Read the model definition and answer for the solid it produces. Units are mm, in the model's axes. A direction names the side the tool comes from. Give positions to 0.01 mm unless a question says otherwise; leave off trailing zeros. Loops run counter-clockwise (first coordinate to the right, second up) from the corner with the lowest first, then second, coordinate; pieces in that order, holes last. Notation, with made-up numbers: (-14.5, 3.5) - (33.5, 3.5) arc R35 ccw to (33.5, 39.5) - close; hole circle Ø7 at (-2.75, -34.5). An arc over 180 degrees is marked (long way). Write item = value, one per line. Start each with the question number.
from build123d import *

# Parameters (mm, degrees)
F1_DEPTH      = 17.5
F1_DEPTH_BACK = 17.5
F2_R          = 2.6
F3_DEPTH      = 10.001
F4_R          = 2.6
F5_DEPTH      = 10.001


with BuildPart() as f1:
    # F0 (on Right) → F1 (new body, two sides)
    with BuildSketch(Plane.YZ) as f1_sk:
        Polygon((-30, 0), (0, 0), (0, 30), (-10, 30), (-10, 10), (-30, 10), align=None)
    extrude(amount=F1_DEPTH)
    extrude(f1_sk.sketch, amount=-F1_DEPTH_BACK)

    # F2 (on face) → F3 (cut, through all)
    with BuildSketch(Plane.XZ.offset(10)):
        with Locations((-7.5, 20)):
            Circle(F2_R)
        with Locations((7.5, 20)):
            Circle(F2_R)
    extrude(amount=-F3_DEPTH, mode=Mode.SUBTRACT)

    # F4 (on face) → F5 (cut, through all)
    with BuildSketch(Plane.XY.offset(10)):
        with Locations((-7.5, -20)):
            Circle(F4_R)
        with Locations((7.5, -20)):
            Circle(F4_R)
    extrude(amount=-F5_DEPTH, mode=Mode.SUBTRACT)


solid = f1.part
1. A cutting plane is placed at B-B on z = 20. Give the vertices of the cut face in (x, y).
2. Given P1, Ø8.5, axis at x = 7.5, y = -20, coming from the +Z side; P2, Ø6, axis at x = 7.5, z = 20, coming from the -Y side, each flat-ended and moving along its own axis, determine where each tip first touches the part or whether it passes through.
3. For a pull along X with two mould halves and no side action, classify faces 1 (the cylindrical face through (-7.838, -5.07, 22.578)), 2 (the flat face through (-17.5, -9, 12)), 3 (the flat face through (0, -5, 30)), 4 (the cylindrical face through (9.98, -19.22, 5.07)) as released by +X, released by -X, zero draft, split by the parting line, or undercut.
4. A cutting plane is placed at C-C on y = -20. Give the vertices of the cut face in (x, z), and give its area (3 significant figures).
5. A cutting plane is placed at A-A on x = 7.5. Give the vertices of the cut face in (y, z), and give its area (3 significant figures).
6. A tool of negligible diameter and unlimited length cuts with its end or side. For faces 5 (the flat face through (0, -20, 10)), 6 (the flat face through (0, 0, 15)), from which of +Z, -Z, +X, -X, +Y, -Y can it reach the whole face along a straight path? Write none if from no direction.
7. Consider line 1 along Z through (x, y) = (12, -11); line 2 along Y through (x, z) = (10, 25.5); line 3 along Z through (x, y) = (-7.5, -7). Determine where each line is inside the solid, lowest interval first. Write a range as [from, to].
8. A cutting plane is placed at D-D on z = 2.5. Give the vertices of the cut face in (x, y), and give its area (3 significant figures).
Reply:
q1.outline = (-17.5, -10) - (-10.1, -10) - (-10.1, 0) - (-17.5, 0) - close; (-4.9, -10) - (4.9, -10) - (4.9, 0) - (-4.9, 0) - close; (10.1, -10) - (17.5, -10) - (17.5, 0) - (10.1, 0) - close
q2.P1 = 10
q2.P2 = -10
q3.face_1 = undercut
q3.face_2 = released by -X
q3.face_3 = zero draft
q3.face_4 = undercut
q4.outline = (-17.5, 0) - (-10.1, 0) - (-10.1, 10) - (-17.5, 10) - close; (-4.9, 0) - (4.9, 0) - (4.9, 10) - (-4.9, 10) - close; (10.1, 0) - (17.5, 0) - (17.5, 10) - (10.1, 10) - close
q4.area = 246 mm^2
q5.outline = (-30, 0) - (-22.6, 0) - (-22.6, 10) - (-30, 10) - close; (-17.4, 0) - (0, 0) - (0, 17.4) - (-10, 17.4) - (-10, 10) - (-17.4, 10) - close; (-10, 22.6) - (0, 22.6) - (0, 30) - (-10, 30) - close
q5.area = 396 mm^2
q6.face_5 = +Z, +X, -X, -Y
q6.face_6 = +Z, -Z, +X, -X, +Y
q7.line_1 = [0, 10]
q7.line_2 = [-10, 0]
q7.line_3 = [0, 17.4], [22.6, 30]
q8.outline = (-17.5, -30) - (17.5, -30) - (17.5, 0) - (-17.5, 0) - close; hole circle Ø5.2 at (-7.5, -20); hole circle Ø5.2 at (7.5, -20)
q8.area = 1,010 mm^2
